from build123d import *

# Parameters (mm, degrees)
SKETCH1_R           = 5
BOSS_EXTRUDE1_DEPTH = 120
SKETCH2_R           = 7
BOSS_EXTRUDE2_DEPTH = 2
FILLET1_R           = 1


with BuildPart() as part:
    # Sketch1 → Boss-Extrude1 (new body)
    with BuildSketch(Plane(origin=(0, 0, 0), x_dir=(1, 0, 0), z_dir=(0, 1, 0))):
        Circle(SKETCH1_R)
    extrude(amount=BOSS_EXTRUDE1_DEPTH)

    # Sketch2 → Boss-Extrude2 (add)
    with BuildSketch(Plane.XZ):
        Circle(SKETCH2_R)
    extrude(amount=BOSS_EXTRUDE2_DEPTH)

    # Fillet1
    fillet1_edges = [part.edges().sort_by_distance(p)[0] for p in [
        (-7, -2, 0),
    ]]
    fillet(fillet1_edges, radius=FILLET1_R)


solid = part.part
For this review, take the finished solid that the model builds, in its own axes (mm). A direction names the side the tool comes from. Give positions to 0.01 mm unless a question says otherwise; leave off trailing zeros. Loops run counter-clockwise (first coordinate to the right, second up) from the corner with the lowest first, then second, coordinate; pieces in that order, holes last. Notation, with made-up numbers: (31, 58.5) -> (53, 58.5) arc R26 cw to (53, 83.5) -> close; hole circle Ø9 at (25, -8.5). An arc over 180 degrees is marked (long way). One line per question, with ' | ' between items.
1) To check wall thickness, follow probe 1 along Y at (x, z) = (5, 2.5); probe 2 along Z at (x, y) = (0, 96). State the ranges of each line that lie inside material, in increasing order.
Resolved:
probe 1: y = -2 to 0 | probe 2: z = -5 to 5
2) We need section B-B (z = 0). Write out the cut boundary in (x, y), plus the area to 3 significant figures.
Resolved:
outline: (-7, -1) arc R1 ccw to (-6, -2) -> (6, -2) arc R1 ccw to (7, -1) -> (7, 0) -> (5, 0) -> (5, 120) -> (-5, 120) -> (-5, 0) -> (-7, 0) -> close | area: 1,230 mm2
3) Insertion check: pin 1 Ø2 at (x, y) = (-4.5, 94) entering from +Z; pin 2 Ø2 at (x, y) = (-0.5, 38) entering from +Z; pin 3 Ø6 at (y, z) = (81, 1) entering from -X. Each pin has a flat end and moves straight along its axis. Give the tip position at first contact, or say it passes through.
Resolved:
pin 1: stops at z = 3.57 | pin 2: stops at z = 5 | pin 3: stops at x = -5
4) For faces 1 (the flat face through (0, 120, 0)), 2 (the cylindrical face through (-1.08, 59.16, 4.88)), list the 3-axis set-ups (+Z, -Z, +X, -X, +Y, -Y) from which the entire face can be reached by the end or side of a thin tool; tool diameter is ignored.
Resolved:
face 1: +Z, -Z, +X, -X, +Y | face 2: +Y
5) We need section A-A (x = 0). Write out the cut boundary in (y, z).
Resolved:
outline: (-2, -6) arc R1 ccw to (-1, -7) -> (0, -7) -> (0, -5) -> (120, -5) -> (120, 5) -> (0, 5) -> (0, 7) -> (-1, 7) arc R1 ccw to (-2, 6) -> close
6) We need section C-C (y = 103). Write out the cut boundary in (x, z).
Resolved:
outline: circle Ø10 at (0, 0)
